Design review of the part built by this model. Coordinates are the model's own, in mm. Coordinates: 2 decimals unless noted, no trailing zeros. Loops run counter-clockwise (first coordinate to the right, second up) from the corner with the lowest first, then second, coordinate; pieces in that order, holes last. Notation, with made-up numbers: (34.25, -7) -> (82.25, -7) arc R29 ccw to (82.25, 27) -> close; hole circle Ø7 at (32.5, 34). An arc over 180 degrees is marked (long way). Use CSV: the item, a comma, the result in double quotes.
```python
from build123d import *

# Parameters (mm, degrees)
F1_DEPTH = 6
F3_DEPTH = 5.9


with BuildPart() as f1:
    # F0 (on Top) → F1 (new body)
    with BuildSketch(Plane.XY):
        with BuildLine():
            ThreePointArc((6, -6), (4.2426406871, -1.7573593129), (0, 0))
            Line((0, 0), (0, -3.4))
            ThreePointArc((0, -3.4), (1.8384776311, -4.1615223689), (2.6, -6))
            ThreePointArc((2.6, -6), (1.8384776311, -7.8384776311), (0, -8.6))
            Line((0, -8.6), (0, -12))
            ThreePointArc((0, -12), (4.2426406871, -10.2426406871), (6, -6))
        make_face()
        with BuildLine():
            Line((0, -3.4), (0, 0))
            ThreePointArc((0, 0), (-6, -6), (0, -12))
            Line((0, -12), (0, -8.6))
            ThreePointArc((0, -8.6), (-2.6, -6), (0, -3.4))
        make_face()
    extrude(amount=F1_DEPTH)

    # F2 (on Front) → F3 (cut)
    with BuildSketch(Plane.XZ):
        with BuildLine():
            ThreePointArc((0, 4.75), (-1.75, 3), (0, 1.25))
            Line((0, 1.25), (0, 4.75))
        make_face()
        with BuildLine():
            Line((0, 4.75), (0, 1.25))
            ThreePointArc((0, 1.25), (1.2374368671, 1.7625631329), (1.75, 3))
            ThreePointArc((1.75, 3), (1.2374368671, 4.2374368671), (0, 4.75))
        make_face()
    extrude(amount=F3_DEPTH, mode=Mode.SUBTRACT)


solid = f1.part
```
Item 1: Add section A-A (x = 2). Give the boundary of the cut face in (y, z).
Checked values:
outline,"(-11.66, 0) -> (-7.66, 0) -> (-7.66, 6) -> (-11.66, 6) -> close; (-4.34, 0) -> (-0.34, 0) -> (-0.34, 6) -> (-4.34, 6) -> close"
Item 2: Add section C-C (y = -3.75). Give the boundary of the cut face in (x, z), then the cut area to 3 significant figures.
Checked values:
outline,"(-5.56, 0) -> (-1.3, 0) -> (-1.3, 1.83) arc R1.75 cw to (-1.3, 4.17) -> (-1.3, 6) -> (-5.56, 6) -> close; (1.3, 0) -> (5.56, 0) -> (5.56, 6) -> (1.3, 6) -> (1.3, 4.17) arc R1.75 cw to (1.3, 1.83) -> close"
area,"49.7 mm^2"
Item 3: Clearance check with flat-ended pins moving along their axes: pin 1 (3 mm diameter, centred on x = -4.5, z = 1, fed in from -Y); pin 2 (1.5 mm diameter, centred on y = -1.5, z = 2.5, fed in from +X); pin 3 (1 mm diameter, centred on x = -1, z = 0.5, fed in from -Y). State where each tip first meets the part, or that it passes through.
Checked values:
pin 1,"y = -11.2"
pin 2,"x = 4.68"
pin 3,"y = -11.98"
Item 4: To check wall thickness, follow line 1 along X through (y, z) = (-2, 1.5); line 2 along Y through (x, z) = (2.25, 0.75); line 3 along Z through (x, y) = (0, -1). State the ranges of each line that lie inside material, in increasing order.
Checked values:
line 1,"-4.47 to -0.9, 0.9 to 4.47"
line 2,"-11.56 to -7.3, -4.7 to -0.44"
line 3,"0 to 1.25, 4.75 to 6"
Item 5: Add section D-D (x = -1.25). Give the boundary of the cut face in (y, z).
Checked values:
outline,"(-11.87, 0) -> (-8.28, 0) -> (-8.28, 6) -> (-11.87, 6) -> close; (-3.72, 0) -> (-0.13, 0) -> (-0.13, 1.78) -> (-3.72, 1.78) -> close; (-3.72, 4.22) -> (-0.13, 4.22) -> (-0.13, 6) -> (-3.72, 6) -> close"
Item 6: Add section B-B (z = 0.5). Give the boundary of the cut face in (x, y).
Checked values:
outline,"circle Ø12 at (0, -6); hole circle Ø5.2 at (0, -6)"
